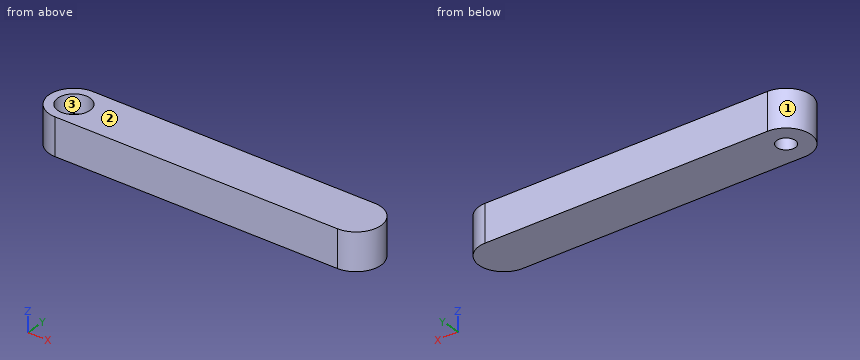
Autodesk Inventor part; units mm, degrees
ref_plane "YZ Plane" through (0, 0, 0) normal (1, 0, 0) x (0, 1, 0)
ref_plane "XZ Plane" through (0, 0, 0) normal (0, 1, 0) x (-1, 0, 0)
ref_plane "XY Plane" through (0, 0, 0) normal (0, 0, 1) x (1, 0, 0)
sketch "Sketch1" plane through (0, 0, 0) normal (0, 0, 1) x (1, 0, 0)
  line L0 (0, 0) -> (46, 0) construction
  line L1 (0, -4) -> (46, -4)
  line L2 (46, 4) -> (0, 4)
  arc A0 (0, 4) -> (0, -4) centre (0, 0) ccw
  arc A1 (46, -4) -> (46, 4) centre (46, 0) ccw
  circle A2 centre (0, 0) radius 1.5
  point P0 (23, 0)
  dimension "d0" = 46
  dimension "d1" = 3
extrude "Extrusion1" add sketch "Sketch1" along normal blind 6
sketch "Sketch2" plane through (0, 0, 6) normal (0, 0, 1) x (1, 0, 0)
  circle A0 centre (0, 0) radius 2.6
  dimension "d4" = 5.2
extrude "Extrusion2" cut sketch "Sketch2" against normal blind 3
properties part number "foot"
Check sheet for the modelled part. Datum: model origin and axes. Units: mm. Face numbers are marked on the shaded views. Round coordinates to 2 decimals unless told otherwise and drop trailing zeros. Write each loop counter-clockwise with the first axis right and the second up, starting at its lowest first coordinate (ties: lowest second). Pieces come first, ordered by that corner, then holes. Notation, with made-up numbers: (56, 20) -> (112, 20) arc R10 ccw to (112, 30) -> close; hole circle Ø2 at (8, 36). An arc over 180 degrees is marked (long way). Answer as CSV lines item,"result". Start each with the question number.
1) Section check A-A on z = 1.4. Enter the section's corners in (x, y), and give its area (3 significant figures).
2) Release check for a two-part mould opening along X. For the marked faces 1, 2 and 3 record: pulls with the +X half, pulls with the -X half, needs draft (parallel to the pull), parting line crosses it, or undercut.
3) Section check B-B on y = 0.75. Enter the section's corners in (x, z), and give its area (3 significant figures).
4) Section check C-C on z = 5. Enter the section's corners in (x, y).
5) Material ranges on line 1 (Y direction, x = 0, z = 1.05); line 2 (Y direction, x = 0, z = 4.2); line 3 (X direction, y = 0, z = 0.75), recorded low to high. Write a range as from..to.
Found:
1,outline,"(0, -4) -> (46, -4) arc R4 ccw to (46, 4) -> (0, 4) arc R4 ccw to start; hole circle Ø3 at (0, 0)"
1,area,"411 mm^2"
2,face 1,"pulls with the -X half"
2,face 2,"needs draft"
2,face 3,"undercut"
3,outline,"(-3.93, 0) -> (-1.3, 0) -> (-1.3, 3) -> (-2.49, 3) -> (-2.49, 6) -> (-3.93, 6) -> close; (1.3, 0) -> (49.93, 0) -> (49.93, 6) -> (2.49, 6) -> (2.49, 3) -> (1.3, 3) -> close"
3,area,"300 mm^2"
4,outline,"(0, -4) -> (46, -4) arc R4 ccw to (46, 4) -> (0, 4) arc R4 ccw to start; hole circle Ø5.2 at (0, 0)"
5,line 1,"y = -4..-1.5, 1.5..4"
5,line 2,"y = -4..-2.6, 2.6..4"
5,line 3,"x = -4..-1.5, 1.5..50"
